from build123d import *

# Parameters (mm, degrees)
F1_DEPTH = 12.7
F2_DEPTH = 31.75
F3_R     = 6.798406
F4_DEPTH = 25.4
F5_SIZE  = 2.54
F7_DEPTH = 31.751


with BuildPart() as f1:
    # F0 (on Top) → F1 (new body)
    with BuildSketch(Plane.XY):
        with BuildLine():
            ThreePointArc((5.042647, -28.126541), (21.916025, -18.336262), (28.575, 0))
            ThreePointArc((28.575, 0), (21.916025, 18.336262), (5.042647, 28.126541))
            ThreePointArc((5.042647, 28.126541), (-28.575, 0), (5.042647, -28.126541))
        make_face()
        with BuildLine():
            ThreePointArc((5.042647, 28.126541), (21.916025, 18.336262), (28.575, 0))
            ThreePointArc((28.575, 0), (21.916025, -18.336262), (5.042647, -28.126541))
            Line((5.042647, -28.126541), (57.336765, -18.751028))
            ThreePointArc((57.336765, -18.751028), (73.025, 0), (57.336765, 18.751028))
            Line((57.336765, 18.751028), (5.042647, 28.126541))
        make_face()
    extrude(amount=F1_DEPTH)

    # F0 (on Top) → F2 (join)
    with BuildSketch(Plane.XY):
        with BuildLine():
            ThreePointArc((5.042647, -28.126541), (21.916025, -18.336262), (28.575, 0))
            ThreePointArc((28.575, 0), (21.916025, 18.336262), (5.042647, 28.126541))
            ThreePointArc((5.042647, 28.126541), (-28.575, 0), (5.042647, -28.126541))
        make_face()
    extrude(amount=F2_DEPTH)

    # F3 (on face) → F4 (cut)
    with BuildSketch(Plane.XY.offset(12.7)):
        with Locations((53.975, 0)):
            Circle(F3_R)
    extrude(amount=-F4_DEPTH, mode=Mode.SUBTRACT)

    # F5
    f5_edges = [f1.edges().sort_by_distance(p)[0] for p in [
        (-5.042647, 28.126541, 31.75),
    ]]
    chamfer(f5_edges, length=F5_SIZE)

    # F6 (on face) → F7 (cut, through all)
    with BuildSketch(Plane.XY.offset(31.75)):
        with BuildLine():
            Line((17.635341, 4.024172), (12.259626, 4.024172))
            ThreePointArc((12.259626, 4.024172), (-12.903193, 0), (12.259626, -4.024172))
            Line((12.259626, -4.024172), (17.635341, -4.024172))
            Line((17.635341, -4.024172), (17.635341, 4.024172))
        make_face()
    extrude(amount=-F7_DEPTH, mode=Mode.SUBTRACT)


solid = f1.part
Geometry check sheet. Reference: the model listing, model coordinates, mm. A direction names the side the tool comes from. Coordinates: 2 decimals unless noted, no trailing zeros. Loops run counter-clockwise (first coordinate to the right, second up) from the corner with the lowest first, then second, coordinate; pieces in that order, holes last. Notation, with made-up numbers: (50.25, 44) - (69.25, 44) arc R8 cw to (69.25, 54) - close; hole circle Ø4 at (-4, 45). An arc over 180 degrees is marked (long way). Use one line per item in the form item = value. Start each with the question number.
Item 1: Mould release check, pull along Y, two halves, no side actions. Record for faces 1 (the face through (22, 0, 0)), 2 (the face through (60.255, -2.604, 6.439)), 3 (the face through (31.556, 23.373, 6.261)): +Y half, -Y half, draft (parallel to the pull), parting line (faces both ways), or undercut.
Item 2: Tool access check on faces 4 (the face through (15, -4.024, 16)), 5 (the face through (30.824, -23.504, 6.261)). Record the directions out of +Z, -Z, +X, -X, +Y, -Y that give a thin tool (end or side, any length) a straight path to the whole face; none if there is none.
Item 3: Section check B-B, the plane x = 37. Enter the section's corners in (y, z).
Item 4: Section check A-A, the plane z = 11. Enter the section's corners in (x, y) (3 decimals).
Item 5: Thickness scan on probe 1 along X at (y, z) = (-1, 11); probe 2 along Y at (x, z) = (0, 14) (3 decimals); probe 3 along Z at (x, y) = (36.5, 13). Record the ranges inside material, lowest first.
Item 6: Gauge pin test, flat ends, axial feed: pin 1 (4 mm diameter, centred on x = 7, y = -5.5, fed in from -Z); pin 2 (5 mm diameter, centred on y = 14, z = 9, fed in from +X); pin 3 (6 mm diameter, centred on y = -13, z = 8.5, fed in from +X); pin 4 (5 mm diameter, centred on x = 38.5, z = 4, fed in from +Y). Record the tip position at first contact, or that the pin passes through.
Computed:
q1.face_1 = draft
q1.face_2 = undercut
q1.face_3 = +Y half
q2.face_4 = +Z, -Z
q2.face_5 = +Z, -Z, +X, -Y
q3.outline = (-22.4, 0) - (22.4, 0) - (22.4, 12.7) - (-22.4, 12.7) - close
q4.outline = (5.043, -28.127) - (57.337, -18.751) arc R19.05 ccw to (57.337, 18.751) - (5.043, 28.127) arc R28.575 ccw (long way) to start; hole (12.26, -4.024) - (17.635, -4.024) - (17.635, 4.024) - (12.26, 4.024) arc R12.903 ccw (long way) to start; hole circle Ø13.597 at (53.975, 0)
q5.probe_1 = -28.56 to -12.86, 17.64 to 47.25, 60.7 to 73
q5.probe_2 = -28.575 to -12.903, 12.903 to 28.575
q5.probe_3 = 0 to 12.7
q6.pin_1 = through
q6.pin_2 = 69.16
q6.pin_3 = 70.19
q6.pin_4 = 22.58
